Autodesk Inventor part; units mm, degrees
ref_plane "YZ Plane" through (0, 0, 0) normal (1, 0, 0) x (0, 1, 0)
ref_plane "XZ Plane" through (0, 0, 0) normal (0, 1, 0) x (-1, 0, 0)
ref_plane "XY Plane" through (0, 0, 0) normal (0, 0, 1) x (1, 0, 0)
sketch "Sketch1" plane through (0, 0, 0) normal (0, 0, 1) x (1, 0, 0)
  line L0 (0, 3.175) -> (2.7496, 1.5875)
  line L1 (2.7496, 1.5875) -> (2.7496, -1.5875)
  line L2 (2.7496, -1.5875) -> (0, -3.175)
  line L3 (0, -3.175) -> (-2.7496, -1.5875)
  line L4 (-2.7496, -1.5875) -> (-2.7496, 1.5875)
  line L5 (-2.7496, 1.5875) -> (0, 3.175)
  point P0 (0, 0)
  point P1 (0, 0)
  dimension "d0" = 6.35
  dimension "d1" = 2.7496
extrude "Extrusion1" add sketch "Sketch1" along normal blind 31.75
sketch "Sketch2" plane through (0, 0, 31.75) normal (0, 0, 1) x (1, 0, 0)
  circle A0 centre (0, 0) radius 4.445
  dimension "d4" = 8.89
extrude "Extrusion2" add sketch "Sketch2" against normal blind 5.08
sketch "Sketch3" plane through (0, 0, 31.75) normal (0, 0, 1) x (1, 0, 0)
  circle A0 centre (0, 0) radius 3.9751 construction
  circle A1 centre (0, 0) radius 2.3813 construction
  line L0 (-5.2785, 0) -> (7.6367, 0) construction
  line L1 (2.0622, 1.1906) -> (3.9751, 0)
  line L2 (3.9751, 0) -> (2.0622, -1.1906)
  line L3 (2.0622, -1.1906) -> (2.0622, 1.1906)
  line L4 (0, 2.3813) -> (1.9876, 3.4425)
  line L5 (1.9876, 3.4425) -> (2.0622, 1.1906)
  line L6 (2.0622, 1.1906) -> (0, 2.3813)
  line L7 (-2.0622, 1.1906) -> (-1.9875, 3.4425)
  line L8 (-1.9875, 3.4425) -> (0, 2.3812)
  line L9 (0, 2.3812) -> (-2.0622, 1.1906)
  line L10 (-2.0622, -1.1906) -> (-3.9751, 0)
  line L11 (-3.9751, 0) -> (-2.0622, 1.1906)
  line L12 (-2.0622, 1.1906) -> (-2.0622, -1.1906)
  line L13 (0, -2.3813) -> (-1.9876, -3.4425)
  line L14 (-1.9876, -3.4425) -> (-2.0622, -1.1906)
  line L15 (-2.0622, -1.1906) -> (0, -2.3813)
  line L16 (2.0622, -1.1906) -> (1.9875, -3.4425)
  line L17 (1.9875, -3.4425) -> (0, -2.3813)
  line L18 (0, -2.3813) -> (2.0622, -1.1906)
  dimension "d7" = 7.9502
  dimension "d8" = 4.7625
  dimension "d9" = 2.0216
  dimension "d10" = 60
  dimension "d11" = 2.3813
  dimension "d14" = 360
extrude "Extrusion3" cut sketch "Sketch3" against normal blind 4.445 contours L1 L2 L3 | L6 L4 L5 | L16 L17 L18 | L9 L7 L8 | L13 L14 L15 | L12 L10 L11
sketch "Sketch4" plane through (0, 0, 31.75) normal (0, 0, 1) x (1, 0, 0)
  line L0 (2.0622, 1.1906) -> (0, 2.3812)
  line L1 (0, 2.3812) -> (-2.0622, 1.1906)
  line L2 (-2.0622, 1.1906) -> (-2.0622, -1.1906)
  line L3 (-2.0622, -1.1906) -> (0, -2.3813)
  line L4 (0, -2.3813) -> (2.0622, -1.1906)
  line L5 (2.0622, -1.1906) -> (2.0622, 1.1906)
  point P0 (0, 0)
extrude "Extrusion4" cut sketch "Sketch4" against normal blind 4.445
properties part number "000111"
For this review, take the finished solid that the model builds, in its own axes (mm). A direction names the side the tool comes from. Coordinates: 2 decimals unless noted, no trailing zeros. Loops run counter-clockwise (first coordinate to the right, second up) from the corner with the lowest first, then second, coordinate; pieces in that order, holes last.
1. Add section C-C, the plane x = 0.5. Give the boundary of the cut face in (y, z) (3 decimals), then the cut area to 3 significant figures.
2. For line 1 (Z direction, x = 0.5, y = 2.5) (3 decimals); line 2 (X direction, y = 0.75, z = 11.5); line 3 (Y direction, x = -2.75, z = 30.5), list the stretches that pass through material, from the lowest coordinate up.
3. For faces 1 (the flat face through (3, 0, 26.67)), 2 (the flat face through (1.36, 2.39, 13.15)), 3 (the flat face through (2.75, 0, 13)), 4 (the flat face through (3.01, 0.6, 29.56)), list the 3-axis set-ups (+Z, -Z, +X, -X, +Y, -Y) from which the entire face can be reached by the end or side of a thin tool; tool diameter is ignored.
4. Mouldability with a two-part tool opening along Y and no side actions: class faces 5 (the flat face through (-1.394, 2.37, 13.148)), 6 (the cylindrical face through (-0.96, -4.34, 29.25)), 7 (the flat face through (-1.36, -2.39, 13.15)), 8 (the flat face through (-3.01, -0.6, 29.56)) as +Y half, -Y half, draft (parallel to the pull), parting line (faces both ways), or undercut.
5. Add section B-B, the plane y = 2. Give the boundary of the cut face in (x, z) (3 decimals).
6. Insertion check: P1, Ø2.5, axis at y = -0.5, z = 12, coming from the +X side; P2, Ø1, axis at x = -3.5, z = 26.5, coming from the +Y side; P3, Ø3.5, axis at y = -0.5, z = 14, coming from the -X side; P4, Ø4, axis at x = -3, y = 0.5, coming from the -Z side. Each pin has a flat end and moves straight along its axis. Give the tip position at first contact, or say it passes through.
7. Add section A-A, the plane z = 12. Give the boundary of the cut face in (x, y) (1 decimal), then the cut area to 3 significant figures.
Result:
1. outline: (-4.417, 26.67) - (-2.886, 26.67) - (-2.886, 0) - (2.886, 0) - (2.886, 26.67) - (4.417, 26.67) - (4.417, 31.75) - (2.648, 31.75) - (2.648, 27.305) - (-2.648, 27.305) - (-2.648, 31.75) - (-4.417, 31.75) - close
1. area: 175 mm2
2. line 1: z = 0 to 27.305
2. line 2: x = -2.75 to 2.75
2. line 3: y = -3.49 to -0.76, 0.76 to 3.49
3. face 1: -Z
3. face 2: -Z, +X, +Y
3. face 3: -Z, +X, +Y, -Y
3. face 4: +Z
4. face 5: +Y half
4. face 6: parting line
4. face 7: -Y half
4. face 8: undercut
5. outline: (-3.97, 26.67) - (-2.035, 26.67) - (-2.035, 0) - (2.035, 0) - (2.035, 26.67) - (3.97, 26.67) - (3.97, 31.75) - (2.035, 31.75) - (2.035, 27.305) - (-2.035, 27.305) - (-2.035, 31.75) - (-3.97, 31.75) - close
6. P1: stops at x = 2.75
6. P2: stops at y = 3.25
6. P3: stops at x = -2.75
6. P4: stops at z = 0
7. outline: (-2.7, -1.6) - (0, -3.2) - (2.7, -1.6) - (2.7, 1.6) - (0, 3.2) - (-2.7, 1.6) - close
7. area: 26.2 mm2
